Geometry: see drawing. Coordinates: mm, zero at the bounding-box minimum. A direction names the side the tool comes from. Round coordinates to 2 decimals unless told otherwise and drop trailing zeros. Loops run counter-clockwise (first coordinate to the right, second up) from the corner with the lowest first, then second, coordinate; pieces in that order, holes last. Notation, with made-up numbers: (18.5, 3) - (58.5, 3) arc R24 cw to (58.5, 18) - close; hole circle Ø5 at (34.25, 49). An arc over 180 degrees is marked (long way). Write item = value, one per line. Start each with the question number.
Item 1: Access query for the marked faces 4 and 5. Directions: +Z, -Z, +X, -X, +Y, -Y. A direction counts if a zero-diameter tool reaches every point of the face in a straight line with its end or side. Return the directions, or none.
Item 2: Line query: line 1 (Y direction, x = 18.5, z = 24); line 2 (Z direction, x = 8.5, y = 21.5); line 3 (Y direction, x = 31.5, z = 13.5). Output: solid intervals per line, ascending. Write a range as from..to.
Item 3: Draft query along Z for the marked faces 1, 2 and 3. Return one class per face: pulls with the +Z half, pulls with the -Z half, needs draft (parallel to the pull), parting line crosses it, or undercut.
Item 4: Section D-D (y = 140). Return loops of the section in (x, z).
Item 5: Section B-B (x = 21). Count the separate pieces of the cut face and the enclosed holes in it, plus the area to 3 significant figures.
Item 6: Section A-A (z = 25). Return loops of the section in (x, y).
Item 7: Section C-C (y = 255). Return loops of the section in (x, z), plus the area to 3 significant figures.
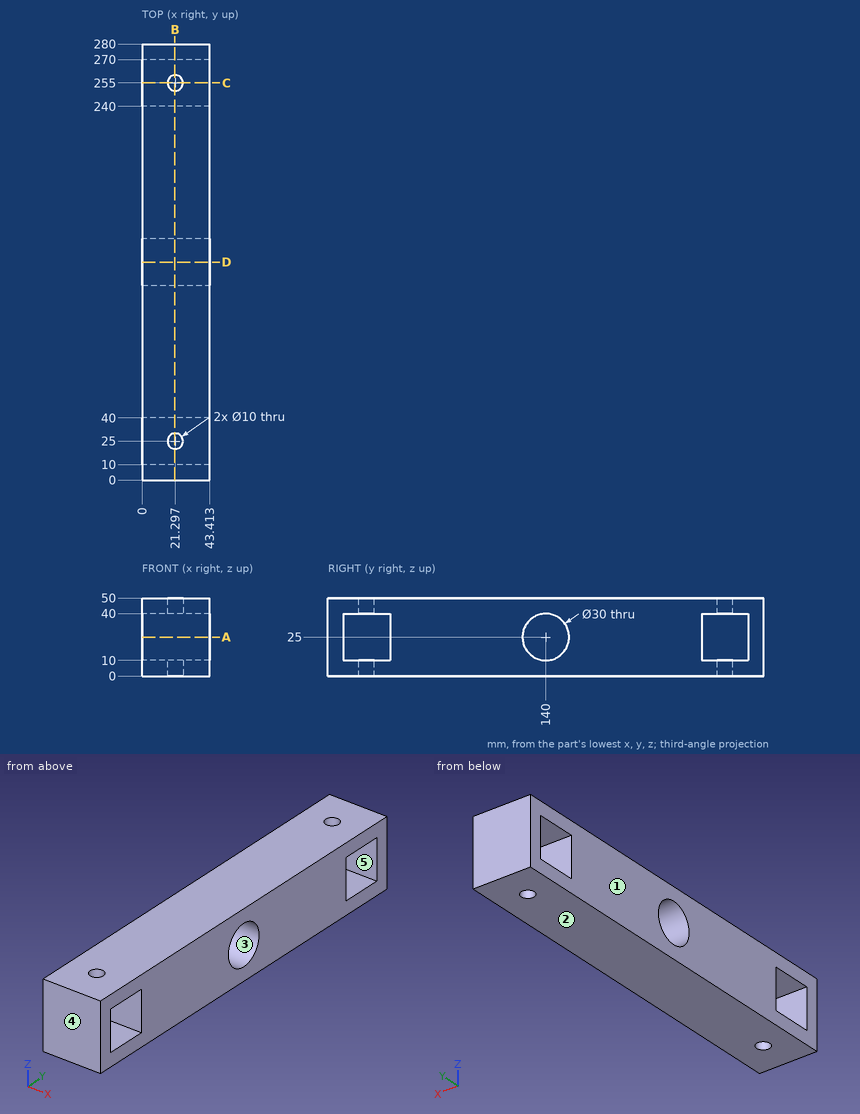
Taken from the geometry:
q1.face_4 = +Z, -Z, +X, -X, -Y
q1.face_5 = +X, -X
q2.line_1 = 0..10, 40..125.03, 154.97..240, 270..280
q2.line_2 = 0..10, 40..50
q2.line_3 = 0..10, 40..130.37, 149.63..240, 270..280
q3.face_1 = needs draft
q3.face_2 = pulls with the -Z half
q3.face_3 = undercut
q4.outline = (0, 0) - (43.41, 0) - (43.41, 10) - (0, 10) - close; (0, 40) - (43.41, 40) - (43.41, 50) - (0, 50) - close
q5.separate_pieces = 3
q5.enclosed_holes = 1
q5.area = 11,100 mm^2
q6.outline = (0, 0) - (43.41, 0) - (43.41, 10) - (0, 10) - close; (0, 40) - (43.41, 40) - (43.41, 125) - (0, 125) - close; (0, 155) - (43.41, 155) - (43.41, 240) - (0, 240) - close; (0, 270) - (43.41, 270) - (43.41, 280) - (0, 280) - close
q7.outline = (0, 0) - (16.3, 0) - (16.3, 10) - (0, 10) - close; (0, 40) - (16.3, 40) - (16.3, 50) - (0, 50) - close; (26.3, 0) - (43.41, 0) - (43.41, 10) - (26.3, 10) - close; (26.3, 40) - (43.41, 40) - (43.41, 50) - (26.3, 50) - close
q7.area = 668 mm^2
